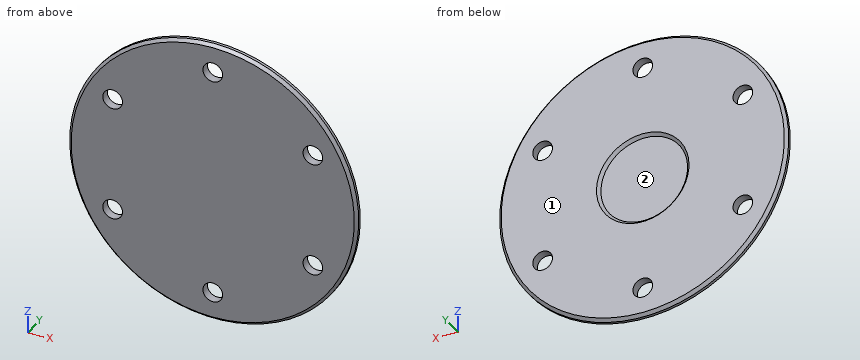
```python
from build123d import *

# Parameters (mm, degrees)
SKETCH_1_R               = 50
EXTRUDE_1_DEPTH          = 3
PATTERN_CIRCULAR_1_COUNT = 6
SKETCH_5_R               = 15
CUT_EXTRUDE_1_DEPTH      = 1
CHAMFER_1_SIZE           = 1


with BuildPart() as part:
    # 草图1 → 凸台-拉伸1 (new body)
    with BuildSketch(Plane(origin=(0, 0, 0), x_dir=(1, 0, 0), z_dir=(0, 1, 0))):
        with Locations(Location((0, 0, 0), (0, 0, 270))):
            Circle(SKETCH_1_R)
    extrude(amount=EXTRUDE_1_DEPTH)

    # 草图4 → M8 螺纹孔的螺纹孔钻头1 (revolve, cut)
    with BuildSketch(Plane(origin=(0, 3, -40), x_dir=(0, 0, 1), z_dir=(1, 0, 0))):
        Polygon((0, 0), (0, 18.042926105), (3.4, 16), (3.4, 0), align=None)
    hole_wizard_m8_1 = revolve(axis=Axis((0, 9.35, -40), (0, -1, 0)), mode=Mode.SUBTRACT)

    # 阵列(圆周)1: M8 螺纹孔的螺纹孔钻头1 ×6 about axis
    pattern_circular_1_axis = Axis((0, 0, 0), (0, 1, 0))
    for i in range(1, PATTERN_CIRCULAR_1_COUNT):
        add(hole_wizard_m8_1.rotate(pattern_circular_1_axis, i * 360 / PATTERN_CIRCULAR_1_COUNT), mode=Mode.SUBTRACT)

    # 草图5 → 切除-拉伸1 (cut)
    with BuildSketch(Plane(origin=(0, 3, 0), x_dir=(1, 0, 0), z_dir=(0, 1, 0))):
        with Locations(Location((0, 0, 0), (0, 0, 270))):
            Circle(SKETCH_5_R)
    extrude(amount=-CUT_EXTRUDE_1_DEPTH, mode=Mode.SUBTRACT)

    # 倒角1
    chamfer_1_edges = [part.edges().sort_by_distance(p)[0] for p in [
        (0, 0, -50),
        (0, 3, -15),
        (0, 3, -50),
    ]]
    chamfer(chamfer_1_edges, length=CHAMFER_1_SIZE - 0.0001)  # a hair under: the kernel refuses the full size


solid = part.part
```
Input: part model. Units: mm. Frame: model coordinates. Face numbers are marked on the shaded views. Give positions to 0.01 mm unless a question says otherwise; leave off trailing zeros. Use a Markdown table: item, result.
(1) Draft query along Z for the marked faces 1 and 2. Return one class per face: released by +Z, released by -Z, zero draft, split by the parting line, or undercut.
Computed values:
| item | result |
|---|---|
| face 1 | zero draft |
| face 2 | undercut |
(2) Section query A-A (x = 0). State how many separate pieces and enclosed holes the cut face has, then the cut area to 3 significant figures.
Computed values:
| item | result |
|---|---|
| separate pieces | 3 |
| enclosed holes | 0 |
| area | 226 mm2 |
(3) Line query: line 1 (X direction, y = 1.75, z = -20); line 2 (Z direction, x = 33.5, y = 2.2); line 3 (X direction, y = 2.35, z = -20). Output: solid intervals per line, ascending. Write a range as from..to.
Computed values:
| item | result |
|---|---|
| line 1 | x = -45.83..-38.04, -31.24..31.24, 38.04..45.83 |
| line 2 | z = -36.85..-23.2, -16.8..16.8, 23.2..36.85 |
| line 3 | x = -45.44..-38.04, -31.24..31.24, 38.04..45.44 |
